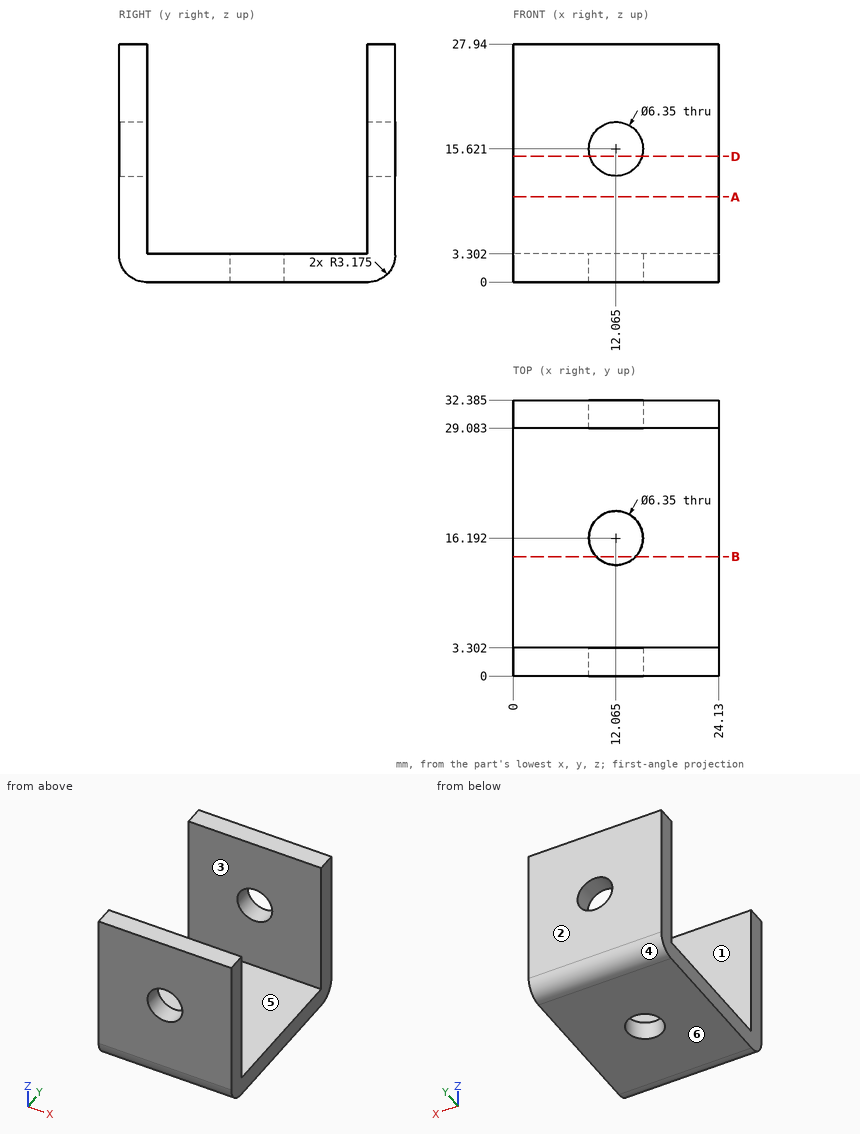
The drawing under review shows one solid part. Ordinate dimensions are in mm from its lowest x, y, z. A direction names the side the tool comes from. Coordinates: 2 decimals unless noted, no trailing zeros. Write each loop counter-clockwise with the first axis right and the second up, starting at its lowest first coordinate (ties: lowest second). Pieces come first, ordered by that corner, then holes. Notation, with made-up numbers: (-21, 76.25) -> (10, 76.25) arc R20 cw to (10, 91.25) -> close; hole circle Ø10 at (6.5, 9). An arc over 180 degrees is marked (long way). One line per item, written item: value. Start each with the question number.
Q1. For the marked faces 1 and 2, list the 3-axis set-ups (+Z, -Z, +X, -X, +Y, -Y) from which the entire face can be reached by the end or side of a thin tool; tool diameter is ignored.
Q2. Clearance check with flat-ended pins moving along their axes: P1, Ø8, axis at x = 10.5, y = 10.5, coming from the +Z side; P2, Ø10, axis at x = 12.065, z = 15.621, coming from the -Y side. State where each tip first meets the part, or that it passes through.
Q3. The part is to be moulded in two halves that separate along Y. For the marked faces 3, 4, 5 and 6, say which applies: +Y half, -Y half, draft (parallel to the pull), parting line (faces both ways), or undercut.
Q4. Add section A-A, the plane z = 10. Give the boundary of the cut face in (x, y) (1 decimal), then the cut area to 3 significant figures.
Q5. To check wall thickness, follow probe 1 along Y at (x, z) = (13.5, 19.5) (1 decimal); probe 2 along Z at (x, y) = (6.75, 25.5); probe 3 along X at (y, z) = (17, 2) (1 decimal). State the ranges of each line that lie inside material, in increasing order.
Q6. Add section B-B, the plane y = 14. Give the boundary of the cut face in (x, z).
Q7. Add section D-D, the plane z = 14.75. Give the boundary of the cut face in (x, y) (1 decimal).
Response:
1. face 1: +Z, +X, -X
1. face 2: +Z, -Z, +X, -X, +Y
2. P1: z = 3.3
2. P2: y = 0
3. face 3: undercut
3. face 4: +Y half
3. face 5: undercut
3. face 6: draft
4. outline: (0, 0) -> (24.1, 0) -> (24.1, 3.3) -> (0, 3.3) -> close; (0, 29.1) -> (24.1, 29.1) -> (24.1, 32.4) -> (0, 32.4) -> close
4. area: 159 mm²
5. probe 1: 0 to 3.3, 29.1 to 32.4
5. probe 2: 0 to 3.3
5. probe 3: 0 to 9, 15.1 to 24.1
6. outline: (0, 0) -> (9.77, 0) -> (9.77, 3.3) -> (0, 3.3) -> close; (14.36, 0) -> (24.13, 0) -> (24.13, 3.3) -> (14.36, 3.3) -> close
7. outline: (0, 0) -> (9, 0) -> (9, 3.3) -> (0, 3.3) -> close; (0, 29.1) -> (9, 29.1) -> (9, 32.4) -> (0, 32.4) -> close; (15.1, 0) -> (24.1, 0) -> (24.1, 3.3) -> (15.1, 3.3) -> close; (15.1, 29.1) -> (24.1, 29.1) -> (24.1, 32.4) -> (15.1, 32.4) -> close
